Could you check a few things on this model? Use its own coordinates, in mm. A direction names the side the tool comes from. Round coordinates to 2 decimals unless told otherwise and drop trailing zeros. Loops run counter-clockwise (first coordinate to the right, second up) from the corner with the lowest first, then second, coordinate; pieces in that order, holes last. Notation, with made-up numbers: (24.25, -38.5) - (52.25, -38.5) arc R20 cw to (52.25, -9.5) - close; hole circle Ø11 at (24, 59.5). An arc over 180 degrees is marked (long way). Use one line per item in the form item = value.
```python
from build123d import *

# Parameters (mm, degrees)
SKETCH2_W           = 35
SKETCH2_H           = 15
SKETCH2_R           = 2
BOSS_EXTRUDE1_DEPTH = 5
BOSS_EXTRUDE6_DEPTH = 15
SKETCH8_R           = 6.25
BOSS_EXTRUDE7_DEPTH = 15
SKETCH10_R          = 2.5
CUT_EXTRUDE1_DEPTH  = 15
CHAMFER1_SIZE       = 0.5


with BuildPart() as part:
    # Sketch2 → Boss-Extrude1 (new body)
    with BuildSketch(Plane(origin=(0, 0, 0), x_dir=(1, 0, 0), z_dir=(0, 1, 0))):
        Rectangle(SKETCH2_W, SKETCH2_H)
        with Locations(Location((-10, 0, 0), (0, 0, 270))):
            Circle(SKETCH2_R, mode=Mode.SUBTRACT)
        with Locations(Location((5, 0, 0), (0, 0, 270))):
            Circle(SKETCH2_R, mode=Mode.SUBTRACT)
    extrude(amount=BOSS_EXTRUDE1_DEPTH)

    # Sketch6 → Boss-Extrude6 (add)
    with BuildSketch(Plane.XY.offset(7.5)):
        with BuildLine():
            Line((17.5, 0), (12.099846669, 0))
            ThreePointArc((12.099846669, 0), (23.57401107, 19.301397513), (40.656768617, 33.874653474))
            ThreePointArc((40.656768617, 33.874653474), (41.649703253, 34.30227285), (42.720886305, 34.44837004))
            Line((42.720886305, 34.44837004), (43, 34.44837004))
            ThreePointArc((43, 34.44837004), (45.828427125, 33.276797165), (47, 30.44837004))
            Line((47, 30.44837004), (47, 7.5))
            Line((47, 7.5), (43, 7.5))
            Line((43, 7.5), (43, 19.677123519))
            ThreePointArc((43, 19.677123519), (40.094264769, 24.217393894), (34.754377969, 23.480534834))
            ThreePointArc((34.754377969, 23.480534834), (24.767284072, 12.739576569), (17.5, 0))
        make_face()
    extrude(amount=-BOSS_EXTRUDE6_DEPTH)

    # Sketch8 → Boss-Extrude7 (add)
    with BuildSketch(Plane.XY.offset(7.5)):
        with Locations((45, 7.5)):
            Circle(SKETCH8_R)
    extrude(amount=-BOSS_EXTRUDE7_DEPTH)

    # Sketch10 → Cut-Extrude1 (cut)
    with BuildSketch(Plane.XY.offset(7.5)):
        with Locations((45, 7.5)):
            Circle(SKETCH10_R)
    extrude(amount=-CUT_EXTRUDE1_DEPTH, mode=Mode.SUBTRACT)

    # Chamfer1
    chamfer1_edges = [part.edges().sort_by_distance(p)[0] for p in [
        (-10, 5, -2),
        (5, 5, -2),
    ]]
    chamfer(chamfer1_edges, length=CHAMFER1_SIZE)


solid = part.part
```
1. If we section it at B-B, the plane x = 5: Write out the boundary of the cut face in (y, z).
Solution:
outline = (0, -7.5) - (5, -7.5) - (5, -2.5) - (4.5, -2) - (0, -2) - close; (0, 2) - (4.5, 2) - (5, 2.5) - (5, 7.5) - (0, 7.5) - close
2. If we section it at A-A, the plane z = 0: Write out the boundary of the cut face in (x, y) (3 decimals).
Solution:
outline = (-17.5, 0) - (-12, 0) - (-12, 4.5) - (-12.5, 5) - (-17.5, 5) - close; (-8, 0) - (3, 0) - (3, 4.5) - (2.5, 5) - (-7.5, 5) - (-8, 4.5) - close; (7, 0) - (17.5, 0) arc R63.733 cw to (34.754, 23.481) arc R5 cw to (43, 19.677) - (43, 13.421) arc R6.25 ccw (long way) to (47, 13.421) - (47, 30.448) arc R4 ccw to (43, 34.448) - (42.721, 34.448) arc R4 ccw to (40.657, 33.875) arc R68.733 ccw to (14.285, 5) - (7.5, 5) - (7, 4.5) - close; hole circle Ø5 at (45, 7.5)
3. On a 3-axis mill with a long thin cutter (end or side, diameter ignored), from which of +Z, -Z, +X, -X, +Y, -Y can I reach the whole of each face in a straight line? I mean faces 4 (the face through (40.17, 24.18, 0.11)), 5 (the face through (24, 12, 7.5)), 6 (the face through (24.889, 12.905, 0.105)), 7 (the face through (47, 22, 0)), 8 (the face through (-2, 5, 0)). Say none if no direction works.
Solution:
face_4 = +Z, -Z
face_5 = +Z, +X, -X, +Y, -Y
face_6 = +Z, -Z, -Y
face_7 = +Z, -Z, +X, +Y
face_8 = +Z, -Z, -X, +Y
4. For P1, Ø5, axis at y = 28.5, z = -1.5, coming from the +X side; P2, Ø3, axis at y = 15, z = -2, coming from the -X side; P3, Ø12, axis at x = 37, y = 18, coming from the -Z side; P4, Ø3.5, axis at x = -10, z = 0, coming from the -Y side, each with a flat end and sliding along its axis, tell me the tip position at first contact or that it passes through.
Solution:
P1 = 47
P2 = 19.19
P3 = -7.5
P4 = through
5. We'd pull the mould along X, two halves only. Please class faces 1 (the face through (45.797, 33.308, 0.105)), 2 (the face through (24, 12, -7.5)), 3 (the face through (43, 17, 0)): +X half, -X half, draft (parallel to the pull), parting line (faces both ways), or undercut.
Solution:
face_1 = +X half
face_2 = draft
face_3 = undercut
6. If we section it at C-C, the plane z = 3.5: Write out the boundary of the cut face in (x, y) (3 decimals), plus the area to 3 significant figures.
Solution:
outline = (-17.5, 0) - (17.5, 0) arc R63.733 cw to (34.754, 23.481) arc R5 cw to (43, 19.677) - (43, 13.421) arc R6.25 ccw (long way) to (47, 13.421) - (47, 30.448) arc R4 ccw to (43, 34.448) - (42.721, 34.448) arc R4 ccw to (40.657, 33.875) arc R68.733 ccw to (14.285, 5) - (-17.5, 5) - close; hole circle Ø5 at (45, 7.5)
area = 577 mm^2
7. Please list where these lines run through material, in increasing order: line 1 along Y through (x, z) = (0.5, -6.5); line 2 along X through (y, z) = (20, -3.5); line 3 along X through (y, z) = (2.4, 0).
Solution:
line_1 = 0 to 5
line_2 = 24.17 to 30.99, 42.99 to 47
line_3 = -17.5 to -12, -8 to 3, 7 to 18.58, 41.39 to 48.61
8. If we section it at D-D, the plane y = 16: Write out the boundary of the cut face in (x, z).
Solution:
outline = (20.96, -7.5) - (27.33, -7.5) - (27.33, 7.5) - (20.96, 7.5) - close; (43, -7.5) - (47, -7.5) - (47, 7.5) - (43, 7.5) - close
